Verification items for this drawing (mm, ordinates from the low corner). A direction names the side the tool comes from. Coordinates: 2 decimals unless noted, no trailing zeros. Loops run counter-clockwise (first coordinate to the right, second up) from the corner with the lowest first, then second, coordinate; pieces in that order, holes last. Notation, with made-up numbers: (46.5, 43.25) - (91.5, 43.25) arc R20 ccw to (91.5, 71.25) - close; hole circle Ø9 at (13.25, 83.25). An arc over 180 degrees is marked (long way). One line per item, written item: value. Start each with the question number.
(1) Section check A-A (y = 6.35). Record the boundary of the cut face in (x, z) (1 decimal), plus the area to 3 significant figures.
(2) Section check D-D (y = 11). Record the boundary of the cut face in (x, z) (1 decimal), plus the area to 3 significant figures.
(3) Thickness scan on probe 1 along X at (y, z) = (6.5, 6.5); probe 2 along X at (y, z) = (12, 1) (1 decimal); probe 3 along X at (y, z) = (6, 2.75) (1 decimal). Record the ranges inside material, lowest first. Write a range as [from, to].
(4) Gauge pin test, flat ends, axial feed: P1, Ø3, axis at x = 22.5, z = 3, coming from the +Y side; P2, Ø1, axis at x = 42, y = 10.5, coming from the -Z side. Record the tip position at first contact, or that the pin passes through.
(5) Set-up check for the marked faces 1 and 2: record each of +Z, -Z, +X, -X, +Y, -Y from which the full face is reachable in a straight line by a thin tool's end or side.
(6) Section check B-B (z = 1). Count the separate pieces of the cut face and the enclosed holes in it, plus the area to 3 significant figures.
(7) Section check C-C (x = 15). Record the boundary of the cut face in (y, z), plus the area to 3 significant figures.
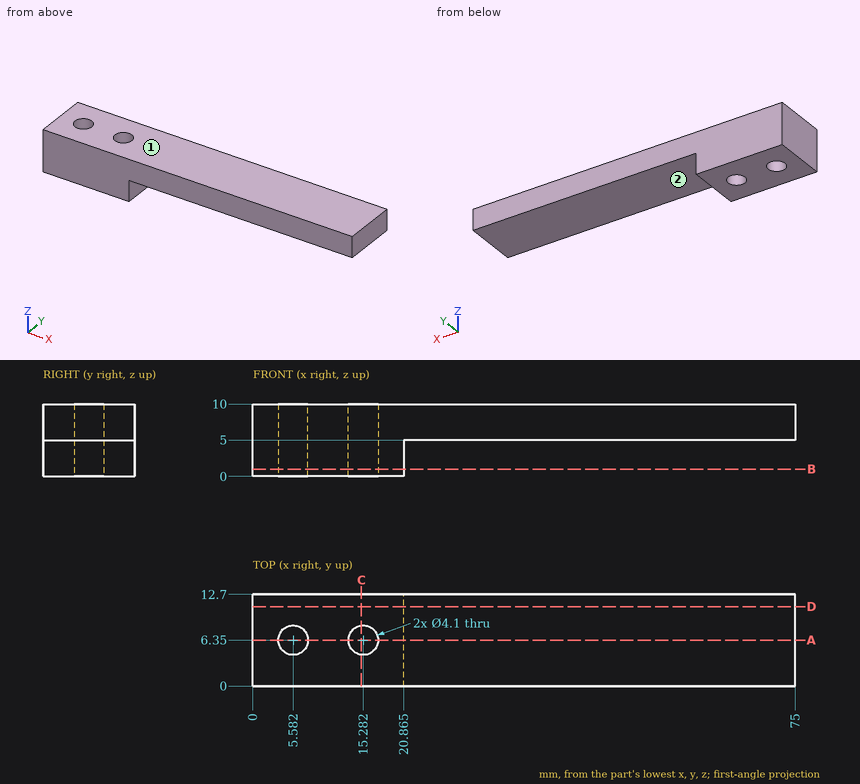
Responses:
1. outline: (0, 0) - (3.5, 0) - (3.5, 10) - (0, 10) - close; (7.6, 0) - (13.2, 0) - (13.2, 10) - (7.6, 10) - close; (17.3, 0) - (20.9, 0) - (20.9, 5) - (75, 5) - (75, 10) - (17.3, 10) - close
1. area: 397 mm²
2. outline: (0, 0) - (20.9, 0) - (20.9, 5) - (75, 5) - (75, 10) - (0, 10) - close
2. area: 479 mm²
3. probe 1: x = [0, 3.54], [7.63, 13.24], [17.33, 75]
3. probe 2: x = [0, 20.9]
3. probe 3: x = [0, 3.6], [7.6, 13.3], [17.3, 20.9]
4. P1: passes through
4. P2: stops at z = 5
5. face 1: +Z, +X, -X, +Y, -Y
5. face 2: -Z, +X, +Y, -Y
6. separate pieces: 1
6. enclosed holes: 2
6. area: 239 mm²
7. outline: (0, 0) - (4.32, 0) - (4.32, 10) - (0, 10) - close; (8.38, 0) - (12.7, 0) - (12.7, 10) - (8.38, 10) - close
7. area: 86.4 mm²
